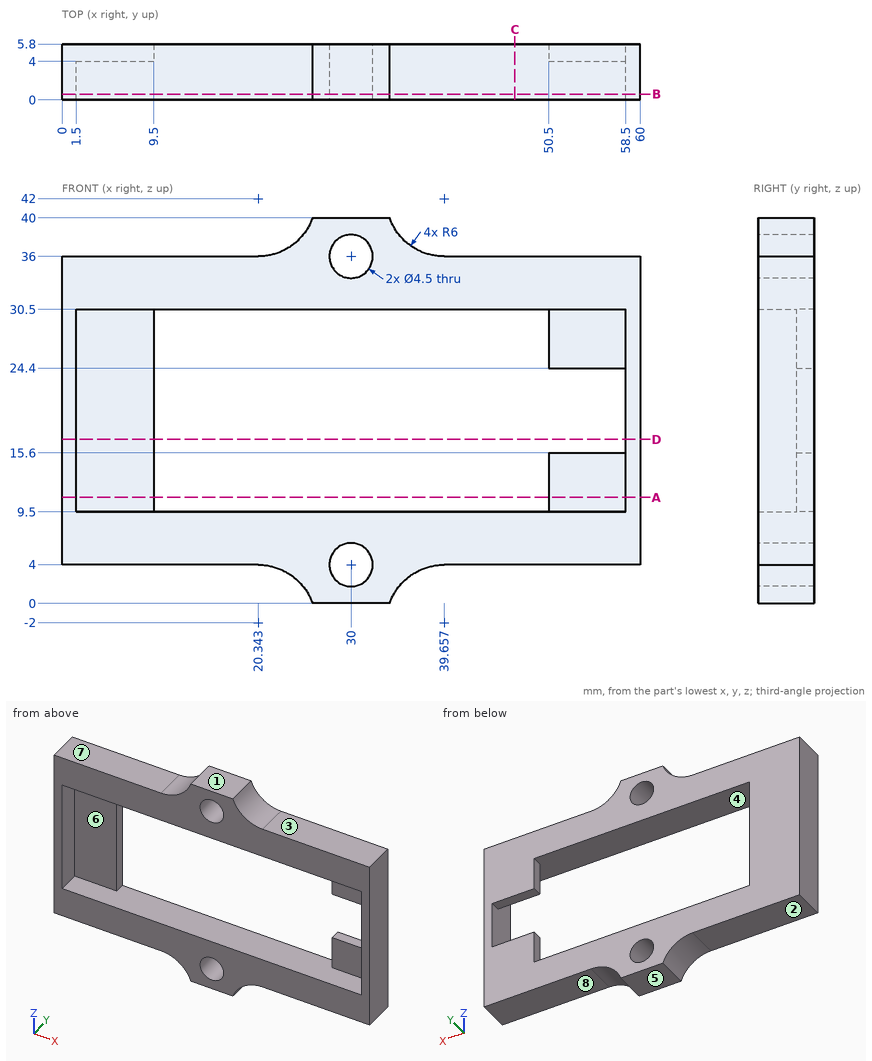
Geometry check sheet. Reference: drawing and pictorial views, mm from the part's lowest x, y, z. A direction names the side the tool comes from. Give positions to 0.01 mm unless a question says otherwise; leave off trailing zeros. Write each loop counter-clockwise with the first axis right and the second up, starting at its lowest first coordinate (ties: lowest second). Pieces come first, ordered by that corner, then holes. Notation, with made-up numbers: (64, 81) - (88, 81) arc R29 cw to (88, 105) - close; hole circle Ø9 at (-16.75, 73.5). An arc over 180 degrees is marked (long way). Put each result on its own line as item: value.
Q1. Mould release check, pull along Z, two halves, no side actions. Record for the marked faces 6, 7 and 8: released by +Z, released by -Z, zero draft, split by the parting line, or undercut.
Result:
face 6: undercut
face 7: released by +Z
face 8: released by -Z
Q2. Set-up check for the marked faces 1, 2, 3, 4 and 5: record each of +Z, -Z, +X, -X, +Y, -Y from which the full face is reachable in a straight line by a thin tool's end or side.
Result:
face 1: +Z, +X, -X, +Y, -Y
face 2: -Z, -X, +Y, -Y
face 3: +Z, +X, +Y, -Y
face 4: -Y
face 5: -Z, +X, -X, +Y, -Y
Q3. Scan lines: probe 1 along Z at (x, y) = (30, 3.6); probe 2 along Z at (x, y) = (13.5, 1.2); probe 3 along X at (y, z) = (5.15, 30). Record each from-to range of solid material in increasing order. Write a range as from..to.
Result:
probe 1: 0..1.75, 6.25..9.5, 30.5..33.75, 38.25..40
probe 2: 4..9.5, 30.5..36
probe 3: 0..9.5, 50.5..60
Q4. Section check A-A on z = 11. Record the cut outline in (x, y).
Result:
outline: (0, 0) - (1.5, 0) - (1.5, 4) - (9.5, 4) - (9.5, 5.8) - (0, 5.8) - close; (50.5, 4) - (58.5, 4) - (58.5, 0) - (60, 0) - (60, 5.8) - (50.5, 5.8) - close
Q5. Section check D-D on z = 17. Record the cut outline in (x, y), and give its area (3 significant figures).
Result:
outline: (0, 0) - (1.5, 0) - (1.5, 4) - (9.5, 4) - (9.5, 5.8) - (0, 5.8) - close; (58.5, 0) - (60, 0) - (60, 5.8) - (58.5, 5.8) - close
area: 31.8 mm2
Q6. Section check B-B on y = 0.6. Record the cut outline in (x, z), and give its area (3 significant figures).
Result:
outline: (0, 4) - (20.34, 4) arc R6 cw to (26, 0) - (34, 0) arc R6 cw to (39.66, 4) - (60, 4) - (60, 36) - (39.66, 36) arc R6 cw to (34, 40) - (26, 40) arc R6 cw to (20.34, 36) - (0, 36) - close; hole (1.5, 9.5) - (58.5, 9.5) - (58.5, 30.5) - (1.5, 30.5) - close; hole circle Ø4.5 at (30, 4); hole circle Ø4.5 at (30, 36)
area: 780 mm2
Q7. Section check C-C on x = 47. Record the cut outline in (y, z).
Result:
outline: (0, 4) - (5.8, 4) - (5.8, 9.5) - (0, 9.5) - close; (0, 30.5) - (5.8, 30.5) - (5.8, 36) - (0, 36) - close
Q8. Depth check by flat-ended pin: P1, Ø1.8, axis at x = 55.5, z = 13, coming from the -Y side; P2, Ø4, axis at x = 19, z = 10, coming from the -Y side; P3, Ø1.7, axis at x = 8.5, y = 2.5, coming from the +Z side; P4, Ø3, axis at x = 5.5, y = 4, coming from the -Z side. Enter the tip coordinate at first touch or a pass-through.
Result:
P1: y = 4
P2: y = 0
P3: z = 36
P4: z = 4
